Check sheet for the modelled part. Datum: model origin and axes. Units: mm. Coordinates: 2 decimals unless noted, no trailing zeros. Write each loop counter-clockwise with the first axis right and the second up, starting at its lowest first coordinate (ties: lowest second). Pieces come first, ordered by that corner, then holes. Notation, with made-up numbers: (69, -13) -> (105, -13) arc R25 ccw to (105, 2) -> close; hole circle Ø5 at (9.5, -28.75). An arc over 180 degrees is marked (long way). One line per item, written item: value. Start each with the question number.
1) Sectioned sample at C-C on x = 0. Enter the section's corners in (y, z).
2) Gauge pin test, flat ends, axial feed: P1, Ø1, axis at x = 7.5, z = 12.5, coming from the +Y side; P2, Ø1.2, axis at x = -7, z = 12.8, coming from the +Y side. Record the tip position at first contact, or that the pin passes through.
3) Sectioned sample at A-A on z = 5.8. Enter the section's corners in (x, y), plus the area to 3 significant figures.
4) Scan lines: line 1 along Z through (x, y) = (0, 2); line 2 along Z through (x, y) = (7, 2.6); line 3 along Z through (x, y) = (0, 0.7). Record each from-to range of solid material in increasing order. Write a range as [from, to].
5) Sectioned sample at B-B on y = 0.8. Enter the section's corners in (x, z), plus the area to 3 significant figures.
6) Sectioned sample at D-D on x = 3. Enter the section's corners in (y, z), plus the area to 3 significant figures.
```python
from build123d import *

# Parameters (mm, degrees)
SKETCH1_W           = 28
SKETCH1_H           = 70.4
BOSS_EXTRUDE1_DEPTH = 3
SKETCH4_R           = 1
CUT_EXTRUDE2_DEPTH  = 10
SKETCH5_R           = 4
CUT_EXTRUDE3_DEPTH  = 10
SKETCH10_R          = 1.75
CUT_EXTRUDE9_DEPTH  = 1.6


with BuildPart() as part:
    # Sketch1 → Boss-Extrude1 (new body)
    with BuildSketch(Plane(origin=(0, 0, 0), x_dir=(1, 0, 0), z_dir=(0, 1, 0))):
        Rectangle(SKETCH1_W, SKETCH1_H)
    extrude(amount=BOSS_EXTRUDE1_DEPTH)

    # Sketch4 → Cut-Extrude2 (cut)
    with BuildSketch(Plane(origin=(0, 3, 0), x_dir=(1, 0, 0), z_dir=(0, 1, 0))):
        with Locations((7, -12.8)):
            Circle(SKETCH4_R)
        with Locations((0, -19.8)):
            Circle(SKETCH4_R)
        with Locations((-7, -12.8)):
            Circle(SKETCH4_R)
        with Locations((0, -5.8)):
            Circle(SKETCH4_R)
    extrude(amount=-CUT_EXTRUDE2_DEPTH, mode=Mode.SUBTRACT)

    # Sketch5 → Cut-Extrude3 (cut)
    with BuildSketch(Plane(origin=(0, 3, 0), x_dir=(1, 0, 0), z_dir=(0, 1, 0))):
        with Locations((0, -12.4)):
            Circle(SKETCH5_R)
    extrude(amount=-CUT_EXTRUDE3_DEPTH, mode=Mode.SUBTRACT)

    # Sketch10 → Cut-Extrude9 (cut)
    with BuildSketch(Plane(origin=(0, 3, 0), x_dir=(1, 0, 0), z_dir=(0, 1, 0))):
        with Locations((0, -19.8)):
            Circle(SKETCH10_R)
        with Locations((-7, -12.8)):
            Circle(SKETCH10_R)
        with Locations((0, -5.8)):
            Circle(SKETCH10_R)
        with Locations((7, -12.8)):
            Circle(SKETCH10_R)
    extrude(amount=-CUT_EXTRUDE9_DEPTH, mode=Mode.SUBTRACT)


solid = part.part
```
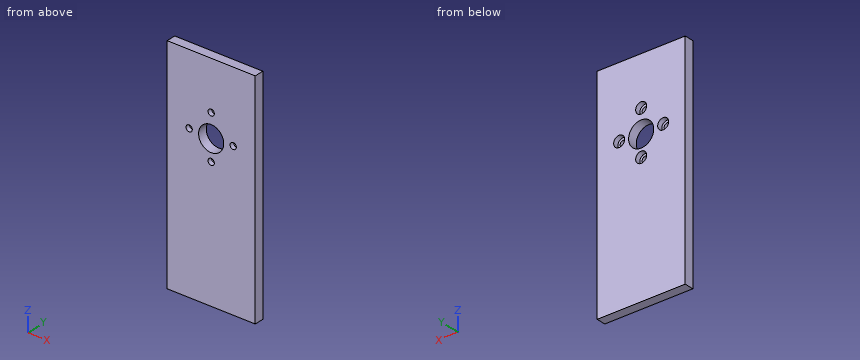
Answers:
1. outline: (0, -35.2) -> (3, -35.2) -> (3, 4.05) -> (1.4, 4.05) -> (1.4, 4.8) -> (0, 4.8) -> close; (0, 6.8) -> (1.4, 6.8) -> (1.4, 7.55) -> (3, 7.55) -> (3, 8.4) -> (0, 8.4) -> close; (0, 16.4) -> (3, 16.4) -> (3, 18.05) -> (1.4, 18.05) -> (1.4, 18.8) -> (0, 18.8) -> close; (0, 20.8) -> (1.4, 20.8) -> (1.4, 21.55) -> (3, 21.55) -> (3, 35.2) -> (0, 35.2) -> close
2. P1: stops at y = 1.4
2. P2: passes through
3. outline: (-14, 0) -> (-1, 0) -> (-1, 1.4) -> (-1.75, 1.4) -> (-1.75, 3) -> (-14, 3) -> close; (1, 0) -> (14, 0) -> (14, 3) -> (1.75, 3) -> (1.75, 1.4) -> (1, 1.4) -> close
3. area: 75.6 mm2
4. line 1: z = [-35.2, 4.05], [7.55, 8.4], [16.4, 18.05], [21.55, 35.2]
4. line 2: z = [-35.2, 11.05], [14.55, 35.2]
4. line 3: z = [-35.2, 4.8], [6.8, 8.4], [16.4, 18.8], [20.8, 35.2]
5. outline: (-14, -35.2) -> (14, -35.2) -> (14, 35.2) -> (-14, 35.2) -> close; hole circle Ø2 at (-7, 12.8); hole circle Ø8 at (0, 12.4); hole circle Ø2 at (0, 5.8); hole circle Ø2 at (0, 19.8); hole circle Ø2 at (7, 12.8)
5. area: 1,910 mm2
6. outline: (0, -35.2) -> (3, -35.2) -> (3, 9.75) -> (0, 9.75) -> close; (0, 15.05) -> (3, 15.05) -> (3, 35.2) -> (0, 35.2) -> close
6. area: 195 mm2
